The model under review builds one solid part; all positions refer to its coordinate system, in mm. A direction names the side the tool comes from. Round coordinates to 2 decimals unless told otherwise and drop trailing zeros. One line per question, with ' | ' between items. Start each with the question number.
```python
from build123d import *

# Parameters (mm, degrees)
F0_W           = 600
F0_H           = 148
F1_DEPTH       = 16
F5_D           = 6.6
F5_CBORE_D     = 11.25
F5_CBORE_DEPTH = 6


with BuildPart() as f1:
    # F0 (on Top) → F1 (new body)
    with BuildSketch(Plane.XY):
        Rectangle(F0_W, F0_H)
    extrude(amount=F1_DEPTH)

    # F5 (through all)
    with Locations(Plane(origin=(0, 0, 0), x_dir=(1, 0, 0), z_dir=(0, 0, -1))):
        with Locations((-109, -52), (-41, -52), (193, 38), (275, 38)):
            CounterBoreHole(F5_D / 2, F5_CBORE_D / 2, F5_CBORE_DEPTH)


solid = f1.part
```
1. Wall thickness on line 1 along X through (y, z) = (52, 11); line 2 along Y through (x, z) = (193, 3.85) (3 decimals); line 3 along X through (y, z) = (52, 3.2) (3 decimals): over which ranges is each line inside the solid? List them lowest first. Write a range as [from, to].
2. The part is to be moulded in two halves that separate along Y. For faces 3 (the face through (-103.635, 50.31, 2.958)), 4 (the face through (-109, 56, 6)), 5 (the face through (-4, 74, 8)), 6 (the face through (-4, 1, 16)), say which applies: pulls with the +Y half, pulls with the -Y half, needs draft (parallel to the pull), parting line crosses it, or undercut.
3. Clearance check with a flat-ended pin moving along its axis: P1, Ø5.5, axis at x = -109.5, y = 53, coming from the -Z side. State where the tip first meets the part, or that it passes through.
4. Machinability: for faces 1 (the face through (192.268, -43.577, 2.958)), 2 (the face through (-4, 1, 0)), which of the approach directions +Z, -Z, +X, -X, +Y, -Y give a long, thin tool a straight path to every point of the face, cutting with its end or side? Answer none if there is none.
Geometry check:
1) line 1: x = [-300, -112.3], [-105.7, -44.3], [-37.7, 300] | line 2: y = [-74, -43.625], [-32.375, 74] | line 3: x = [-300, -114.625], [-103.375, -46.625], [-35.375, 300]
2) face 3: undercut | face 4: undercut | face 5: pulls with the +Y half | face 6: needs draft
3) P1: stops at z = 6
4) face 1: -Z | face 2: -Z, +X, -X, +Y, -Y
